Can you work these out from the model? Positions are in its coordinate system, mm. A direction names the side the tool comes from. Give positions to 0.01 mm unless a question says otherwise; leave off trailing zeros. Order: outer loops, then holes, each group sorted by start corner. A loop starts at its lowest first (then second) coordinate and runs counter-clockwise, first axis right, second up. Notation, with made-up numbers: (-34.5, -19) - (23.5, -19) arc R20 cw to (23.5, -14) - close; hole circle Ø9 at (26, -28). An arc over 180 degrees is marked (long way). Answer as a JSON object with one key per item and string values.
```python
from build123d import *

# Parameters (mm, degrees)
BOSS_EXTRUDE1_DEPTH = 180
CUT_EXTRUDE1_DEPTH  = 3


with BuildPart() as part:
    # Sketch1 → Boss-Extrude1 (new body)
    with BuildSketch(Plane.XY):
        Polygon((-79.798311646, 0.218218313), (-80.70225823, -2.265354514), (73.635788627, -2.265354514), (72.731842043, 0.218218313), (72.700720755, 0.303723349), (72.541884773, 0.303723349), (-79.767190358, 0.303723349), align=None)
    extrude(amount=-BOSS_EXTRUDE1_DEPTH)

    # Sketch2 → Cut-Extrude1 (cut)
    with BuildSketch(Plane(origin=(0, 0.303723349, 0), x_dir=(1, 0, 0), z_dir=(0, 1, 0))):
        with BuildLine():
            Line((-41.65021258, 50), (34.583742977, 50))
            ThreePointArc((34.583742977, 50), (39.583742977, 45), (34.583742977, 40))
            Line((34.583742977, 40), (-41.65021258, 40))
            ThreePointArc((-41.65021258, 40), (-46.65021258, 45), (-41.65021258, 50))
        make_face()
        with BuildLine():
            Line((-56.99562327, 30.024566053), (51.503813463, 30.024566053))
            ThreePointArc((51.503813463, 30.024566053), (56.503813463, 25.024566053), (51.503813463, 20.024566053))
            Line((51.503813463, 20.024566053), (-58.570283066, 20.024566053))
            ThreePointArc((-58.570283066, 20.024566053), (-63.570283066, 25.024566053), (-58.570283066, 30.024566053))
            Line((-58.570283066, 30.024566053), (-56.99562327, 30.024566053))
        make_face()
        with BuildLine():
            Line((-56.99562327, 149.975433947), (-58.570283066, 149.975433947))
            ThreePointArc((-58.570283066, 149.975433947), (-63.570283066, 154.975433947), (-58.570283066, 159.975433947))
            Line((-58.570283066, 159.975433947), (51.503813463, 159.975433947))
            ThreePointArc((51.503813463, 159.975433947), (56.503813463, 154.975433947), (51.503813463, 149.975433947))
            Line((51.503813463, 149.975433947), (-56.99562327, 149.975433947))
        make_face()
        with BuildLine():
            Line((-41.65021258, 140), (34.583742977, 140))
            ThreePointArc((34.583742977, 140), (39.583742977, 135), (34.583742977, 130))
            Line((34.583742977, 130), (-41.65021258, 130))
            ThreePointArc((-41.65021258, 130), (-46.65021258, 135), (-41.65021258, 140))
        make_face()
    extrude(amount=-CUT_EXTRUDE1_DEPTH, mode=Mode.SUBTRACT)


solid = part.part
```
Q1. I need wall thicknesses on L1, parallel to Z at x = 33.5, y = 0.1; L2, parallel to Z at x = 46, y = -0.6; L3, parallel to Z at x = 56, y = 0. Which ranges of each line are inside material? Lowest first, please.
Recorded:
{"L1": "z = -180 to -159.98, -149.98 to -140, -130 to -50, -40 to -30.02, -20.02 to 0", "L2": "z = -180 to -159.98, -149.98 to -30.02, -20.02 to 0", "L3": "z = -180 to -157.16, -152.79 to -27.21, -22.84 to 0"}
Q2. I'm going to push flat-ended pins straight in: pin 1 Ø1.5 at (x, y) = (54, -1) entering from +Z; pin 2 Ø4 at (x, z) = (-43.5, -43.5) entering from -Y. Where does each tip first touch, or does it pass through?
Recorded:
{"pin 1": "stops at z = 0", "pin 2": "passes through"}
Q3. Which directions (+Z, -Z, +X, -X, +Y, -Y) give clear straight access to the entire face, cutting with the end or side of a thin tool? Please do faces 1 (the face through (-2, 0.304, -89)), 2 (the face through (39.583, -0.963, -45.11)).
Recorded:
{"face 1": "+Z, -Z, +X, -X, +Y", "face 2": "+Y, -Y"}
Q4. If we section it at C-C, the plane y = -1.7: Please give me the cut outline in (x, z).
Recorded:
{"outline": "(-80.5, -180) - (73.43, -180) - (73.43, 0) - (-80.5, 0) - close; hole (-58.57, -159.98) - (51.5, -159.98) arc R5 ccw to (51.5, -149.98) - (-58.57, -149.98) arc R5 ccw to start; hole (-58.57, -30.02) - (51.5, -30.02) arc R5 ccw to (51.5, -20.02) - (-58.57, -20.02) arc R5 ccw to start; hole (-41.65, -140) - (34.58, -140) arc R5 ccw to (34.58, -130) - (-41.65, -130) arc R5 ccw to start; hole (-41.65, -50) - (34.58, -50) arc R5 ccw to (34.58, -40) - (-41.65, -40) arc R5 ccw to start"}
Q5. If we section it at A-A, the plane z = -135: Please give me the cut outline in (x, y), then the cut area to 3 significant figures.
Recorded:
{"outline": "(-80.7, -2.27) - (-46.65, -2.27) - (-46.65, 0.3) - (-79.77, 0.3) - close; (39.58, -2.27) - (73.64, -2.27) - (72.7, 0.3) - (39.58, 0.3) - close", "area": "173 mm^2"}
Q6. If we section it at B-B, the plane x = -28: Please give me the cut outline in (y, z).
Recorded:
{"outline": "(-2.27, -180) - (0.3, -180) - (0.3, -159.98) - (-2.27, -159.98) - close; (-2.27, -149.98) - (0.3, -149.98) - (0.3, -140) - (-2.27, -140) - close; (-2.27, -130) - (0.3, -130) - (0.3, -50) - (-2.27, -50) - close; (-2.27, -40) - (0.3, -40) - (0.3, -30.02) - (-2.27, -30.02) - close; (-2.27, -20.02) - (0.3, -20.02) - (0.3, 0) - (-2.27, 0) - close"}
